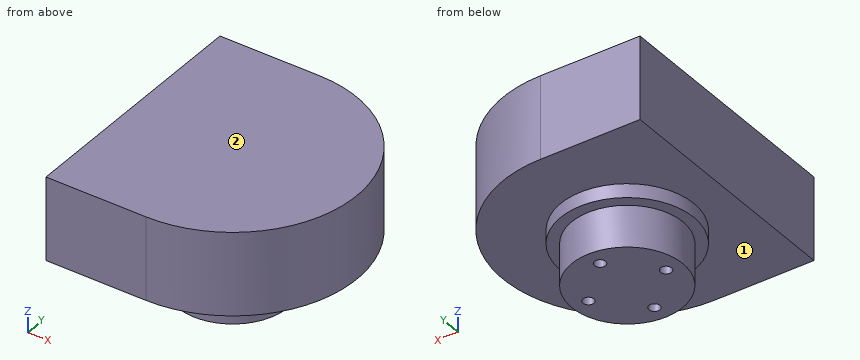
```python
from build123d import *

# Parameters (mm, degrees)
SKETCH_1_W          = 189.06
SKETCH_1_H          = 44.73
EXTRUDE_1_DEPTH     = 15
CUT_EXTRUDE_4_REACH = 196.858
SKETCH_6_R          = 10
EXTRUDE_2_DEPTH     = 10
SKETCH_7_R          = 1
CUT_EXTRUDE_6_DEPTH = 5
SKETCH_8_R          = 12
SKETCH_8_R_2        = 10
EXTRUDE_3_DEPTH     = 2.5


with BuildPart() as part:
    # 草图1 → 凸台-拉伸1 (new body)
    with BuildSketch(Plane.XY):
        with Locations((94.53, 22.365)):
            Rectangle(SKETCH_1_W, SKETCH_1_H)
    extrude(amount=EXTRUDE_1_DEPTH)

    # 草图4 → 切除-拉伸4 (cut, up to next)
    with BuildSketch(Plane.XY.offset(15), mode=Mode.PRIVATE) as cut_extrude_4_sk1:
        with BuildLine():
            Line((189.06, 44.73), (18, 44.73))
            ThreePointArc((18, 44.73), (40.365, 22.365), (18, 0))
            Line((18, 0), (189.06, 0))
            Line((189.06, 0), (189.06, 44.73))
        make_face()
    cut_extrude_4_tool1 = extrude(cut_extrude_4_sk1.sketch, amount=-CUT_EXTRUDE_4_REACH, mode=Mode.PRIVATE) & part.part
    add(cut_extrude_4_tool1.solids().sort_by_distance((112.231547, 22.365, 15))[0], mode=Mode.SUBTRACT)

    # 草图6 → 凸台-拉伸2 (add)
    with BuildSketch(Plane(origin=(0, 0, 0), x_dir=(-1, 0, 0), z_dir=(0, 0, -1))):
        with Locations((-18, 22.365)):
            Circle(SKETCH_6_R)
    extrude(amount=EXTRUDE_2_DEPTH)

    # 草图7 → 切除-拉伸6 (cut)
    with BuildSketch(Plane(origin=(0, 0, -10), x_dir=(-1, 0, 0), z_dir=(0, 0, -1))):
        with Locations((-18, 29.365)):
            Circle(SKETCH_7_R)
        with Locations((-11, 22.365)):
            Circle(SKETCH_7_R)
        with Locations((-18, 15.365)):
            Circle(SKETCH_7_R)
        with Locations((-25, 22.365)):
            Circle(SKETCH_7_R)
    extrude(amount=-CUT_EXTRUDE_6_DEPTH, mode=Mode.SUBTRACT)

    # 草图8 → 凸台-拉伸3 (add)
    with BuildSketch(Plane(origin=(0, 0, 0), x_dir=(-1, 0, 0), z_dir=(0, 0, -1))):
        with Locations((-18, 22.365)):
            Circle(SKETCH_8_R)
        with Locations((-18, 22.365)):
            Circle(SKETCH_8_R_2, mode=Mode.SUBTRACT)
    extrude(amount=EXTRUDE_3_DEPTH)


solid = part.part
```
Part model, mm, in its own coordinate system. Face numbers are marked on the shaded views. A direction names the side the tool comes from. Round coordinates to 2 decimals unless told otherwise and drop trailing zeros. Loops run counter-clockwise (first coordinate to the right, second up) from the corner with the lowest first, then second, coordinate; pieces in that order, holes last. Notation, with made-up numbers: (51, -15.75) -> (74, -15.75) arc R13 cw to (74, 5.25) -> close; hole circle Ø5 at (62.5, -16). An arc over 180 degrees is marked (long way). Use CSV: the item, a comma, the result in double quotes. Start each with the question number.
1) Cut at D-D, the plane x = 15.5. Write the cut outline in (y, z).
2) Cut at B-B, the plane y = 27. Write the cut outline in (x, z).
3) Which spindle directions (+Z, -Z, +X, -X, +Y, -Y) get a long thin tool onto all of the face, cutting with end or side? Do the marked faces 1 and 2. Say none if no direction does.
4) Cut at C-C, the plane z = 8. Write the cut outline in (x, y) (3 decimals), plus the area to 3 significant figures.
5) Wall check: L1, parallel to Y at x = 18, z = -6.4 (3 decimals); L2, parallel to Z at x = 29, y = 3; L3, parallel to Y at x = 25, z = -8.55 (3 decimals). Give the ranges that are in metal, low to high. Write a range as [from, to].
6) Cut at A-A, the plane x = 25. Write the cut outline in (y, z) (3 decimals).
7) Drop flat-ended pins along their axis: P1, Ø0.6, axis at x = 11.5, y = 22.5, coming from the -Z side; P2, Ø1.5, axis at x = 30, y = 36, coming from the -Z side; P3, Ø10, axis at y = 22, z = 7.5, coming from the +X side (3 decimals). Give the stop position or say it passes through.
Determined:
1,outline,"(0, 0) -> (10.63, 0) -> (10.63, -2.5) -> (12.68, -2.5) -> (12.68, -10) -> (32.05, -10) -> (32.05, -2.5) -> (34.1, -2.5) -> (34.1, 0) -> (44.73, 0) -> (44.73, 15) -> (0, 15) -> close"
2,outline,"(0, 0) -> (6.93, 0) -> (6.93, -2.5) -> (9.14, -2.5) -> (9.14, -10) -> (26.86, -10) -> (26.86, -2.5) -> (29.07, -2.5) -> (29.07, 0) -> (39.88, 0) -> (39.88, 15) -> (0, 15) -> close"
3,face 1,"-Z"
3,face 2,"+Z, +X, -X, +Y, -Y"
4,outline,"(0, 0) -> (18, 0) arc R22.365 ccw to (18, 44.73) -> (0, 44.73) -> close"
4,area,"1,590 mm2"
5,L1,"y = [12.365, 14.365], [16.365, 28.365], [30.365, 32.365]"
5,L2,"z = [0, 15]"
5,L3,"y = [15.224, 21.365], [23.365, 29.506]"
6,outline,"(1.124, 0) -> (12.618, 0) -> (12.618, -2.5) -> (15.224, -2.5) -> (15.224, -10) -> (21.365, -10) -> (21.365, -5) -> (23.365, -5) -> (23.365, -10) -> (29.506, -10) -> (29.506, -2.5) -> (32.112, -2.5) -> (32.112, 0) -> (43.606, 0) -> (43.606, 15) -> (1.124, 15) -> close"
7,P1,"stops at z = -5"
7,P2,"stops at z = 0"
7,P3,"stops at x = 40.365"
